```python
from build123d import *

# Parameters (mm, degrees)
SKETCH1_W           = 32
SKETCH1_H           = 32
BOSS_EXTRUDE1_DEPTH = 1.75
CHAMFER1_SIZE       = 7


with BuildPart() as part:
    # Sketch1 → Boss-Extrude1 (new body)
    with BuildSketch(Plane(origin=(0, 0, 0), x_dir=(1, 0, 0), z_dir=(0, 1, 0))):
        Rectangle(SKETCH1_W, SKETCH1_H)
    extrude(amount=-BOSS_EXTRUDE1_DEPTH)

    # Chamfer1
    chamfer1_edges = [part.edges().sort_by_distance(p)[0] for p in [
        (16, -0.875, 16),
        (-16, -0.875, 16),
        (-16, -0.875, -16),
        (16, -0.875, -16),
    ]]
    chamfer(chamfer1_edges, length=CHAMFER1_SIZE)


solid = part.part
```
Part model, mm, in its own coordinate system. Round coordinates to 2 decimals unless told otherwise and drop trailing zeros. Write each loop counter-clockwise with the first axis right and the second up, starting at its lowest first coordinate (ties: lowest second). Pieces come first, ordered by that corner, then holes. Notation, with made-up numbers: (-2.5, 66) -> (42.5, 66) arc R23 ccw to (42.5, 88) -> close; hole circle Ø3 at (-15.75, -23). An arc over 180 degrees is marked (long way). Return JSON: item names as keys, results as strings. Group by question number.
Q1. Saw through at A-A on y = -0.8. Write the cut outline in (x, z), plus the area to 3 significant figures.
Q2. Saw through at C-C on x = -10. Write the cut outline in (y, z).
Q3. Probe L1, parallel to X at y = -1.3, z = -14; L2, parallel to X at y = -0.5, z = 13; L3, parallel to Z at x = 13.5, y = -0.3. List the from-to ranges inside material, lowest first. Write a range as [from, to].
Q4. Saw through at B-B on z = 12. Write the cut outline in (x, y), plus the area to 3 significant figures.
Answer:
{
 "1": {"outline": "(-16, -9) -> (-9, -16) -> (9, -16) -> (16, -9) -> (16, 9) -> (9, 16) -> (-9, 16) -> (-16, 9) -> close", "area": "926 mm2"},
 "2": {"outline": "(-1.75, -15) -> (0, -15) -> (0, 15) -> (-1.75, 15) -> close"},
 "3": {"L1": "[-11, 11]", "L2": "[-12, 12]", "L3": "[-11.5, 11.5]"},
 "4": {"outline": "(-13, -1.75) -> (13, -1.75) -> (13, 0) -> (-13, 0) -> close", "area": "45.5 mm2"}
}
